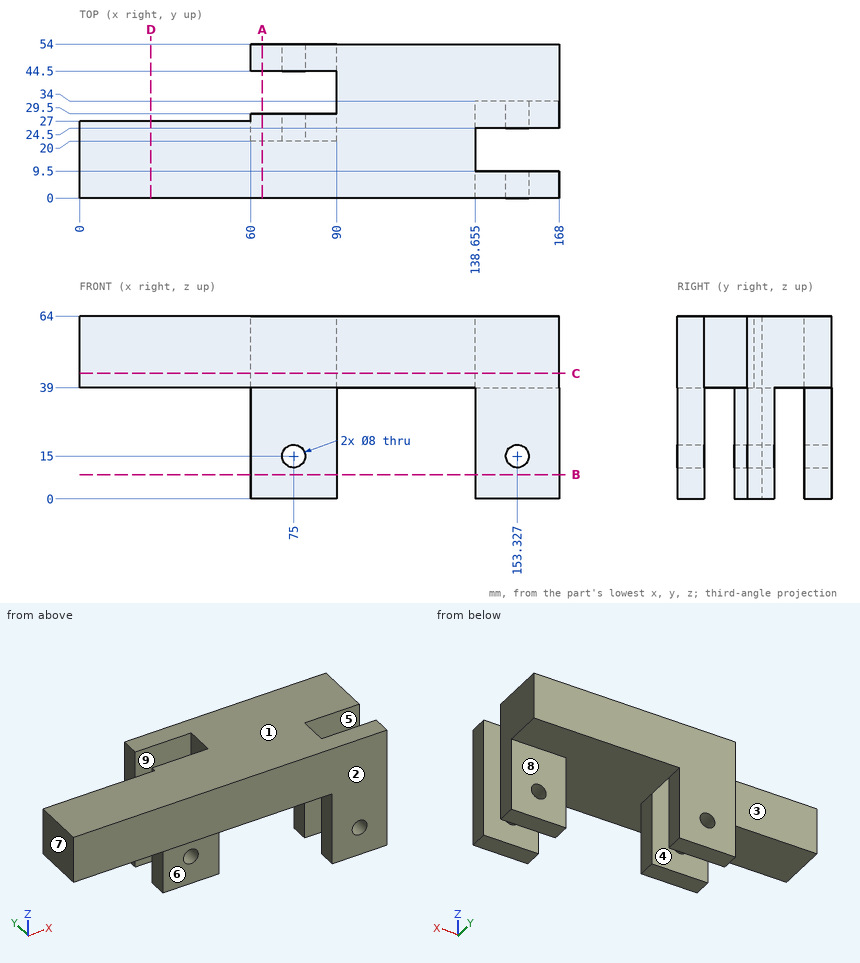
Design review of the part shown in the three views and the two pictorial views. Dimensions are in mm from the part's minimum x, y and z. A direction names the side the tool comes from. Coordinates: 2 decimals unless noted, no trailing zeros. Write each loop counter-clockwise with the first axis right and the second up, starting at its lowest first coordinate (ties: lowest second). Pieces come first, ordered by that corner, then holes. Notation, with made-up numbers: (72.25, 33.5) -> (123.25, 33.5) arc R5 ccw to (123.25, 39.5) -> close; hole circle Ø8 at (7, 50). An arc over 180 degrees is marked (long way). Answer in a Markdown table with one row per item.
1. We need section C-C, the plane z = 44. State the section outline as (x, y) points (1 decimal), and give its area (3 significant figures).
Answers below:
| item | result |
|---|---|
| outline | (0, 0) -> (168, 0) -> (168, 9.5) -> (138.7, 9.5) -> (138.7, 24.5) -> (168, 24.5) -> (168, 54) -> (60, 54) -> (60, 44.5) -> (90, 44.5) -> (90, 29.5) -> (60, 29.5) -> (60, 27) -> (0, 27) -> close |
| area | 6,560 mm^2 |
2. Draft analysis for pull direction Y (two halves, no side actions). For the marked faces 1, 2, 3 and 4, state which applies: +Y half, -Y half, draft (parallel to the pull), parting line (faces both ways), or undercut.
Answers below:
| item | result |
|---|---|
| face 1 | draft |
| face 2 | -Y half |
| face 3 | +Y half |
| face 4 | undercut |
3. We need section D-D, the plane x = 25. State the section outline as (y, z) points, and give its area (3 significant figures).
Answers below:
| item | result |
|---|---|
| outline | (0, 39) -> (27, 39) -> (27, 64) -> (0, 64) -> close |
| area | 675 mm^2 |
4. Clearance check with flat-ended pins moving along their axes: pin 1 Ø4.5 at (y, z) = (19, 57) entering from +X (1 decimal); pin 2 Ø10 at (y, z) = (28.5, 29) entering from -X; pin 3 Ø12 at (y, z) = (37.5, 50.5) entering from -X. State where each tip first meets the part, or that it passes through.
Answers below:
| item | result |
|---|---|
| pin 1 | stops at x = 138.7 |
| pin 2 | stops at x = 60 |
| pin 3 | stops at x = 90 |
5. Wall thickness on probe 1 along X at (y, z) = (26, 15) (1 decimal); probe 2 along Y at (x, z) = (79.5, 33.5); probe 3 along Y at (x, z) = (151, 26): over which ranges is each line inside the solid? List them lowest first. Write a range as [from, to].
Answers below:
| item | result |
|---|---|
| probe 1 | x = [60, 71], [79, 90], [138.7, 149.3], [157.3, 168] |
| probe 2 | y = [20, 29.5], [44.5, 54] |
| probe 3 | y = [0, 9.5], [24.5, 34] |
6. For the marked faces 5, 6, 7, 8 and 9, list the 3-axis set-ups (+Z, -Z, +X, -X, +Y, -Y) from which the entire face can be reached by the end or side of a thin tool; tool diameter is ignored.
Answers below:
| item | result |
|---|---|
| face 5 | +Z, -Z, +X |
| face 6 | -Z, +X, -X, -Y |
| face 7 | +Z, -Z, -X, +Y, -Y |
| face 8 | -Z, +X, -X, +Y |
| face 9 | +Z, -Z, -X |
7. We need section A-A, the plane x = 64. State the section outline as (y, z) points, and give its area (3 significant figures).
Answers below:
| item | result |
|---|---|
| outline | (0, 39) -> (20, 39) -> (20, 0) -> (29.5, 0) -> (29.5, 64) -> (0, 64) -> close; (44.5, 0) -> (54, 0) -> (54, 64) -> (44.5, 64) -> close |
| area | 1,720 mm^2 |
8. We need section B-B, the plane z = 8.5. State the section outline as (x, y) points (1 decimal), and give its area (3 significant figures).
Answers below:
| item | result |
|---|---|
| outline | (60, 20) -> (90, 20) -> (90, 29.5) -> (60, 29.5) -> close; (60, 44.5) -> (90, 44.5) -> (90, 54) -> (60, 54) -> close; (138.7, 0) -> (168, 0) -> (168, 9.5) -> (138.7, 9.5) -> close; (138.7, 24.5) -> (168, 24.5) -> (168, 34) -> (138.7, 34) -> close |
| area | 1,130 mm^2 |
